from build123d import *

# Parameters (mm, degrees)
F1_DEPTH = 25.4
F2_T     = -5.08
F3_SIZE  = 10.16
F4_R     = 10.16
F5_R     = 15.875
F6_DEPTH = 25.4


with BuildPart() as f1:
    # F0 (on Top) → F1 (new body)
    with BuildSketch(Plane.XY):
        Polygon((25.4, 43.9940905122), (-25.4, 43.9940905122), (-50.8, 0), (-25.4, -43.9940905122), (25.4, -43.9940905122), (50.8, 0), align=None)
    extrude(amount=F1_DEPTH)

    # F2
    f2_openings = [f1.faces().sort_by_distance(p)[0] for p in [
        (0, 0, 25.4),
    ]]
    offset(amount=F2_T, openings=f2_openings)

    # F3
    f3_edges = [f1.edges().sort_by_distance(p)[0] for p in [
        (0, 38.914091, 5.08),
        (33.700591, 19.457045, 5.08),
        (-33.700591, 19.457045, 5.08),
        (-33.700591, -19.457045, 5.08),
        (0, -38.914091, 5.08),
        (33.700591, -19.457045, 5.08),
    ]]
    chamfer(f3_edges, length=F3_SIZE)

    # F4
    f4_edges = [f1.edges().sort_by_distance(p)[0] for p in [
        (0, 28.754091, 5.08),
        (24.901773, 14.377045, 5.08),
        (-24.901773, 14.377045, 5.08),
        (24.901773, -14.377045, 5.08),
        (-24.901773, -14.377045, 5.08),
        (0, -28.754091, 5.08),
    ]]
    fillet(f4_edges, radius=F4_R)

    # F5 (on face) → F6 (cut)
    with BuildSketch(Plane.XY.offset(5.08)):
        Circle(F5_R)
    extrude(amount=-F6_DEPTH, mode=Mode.SUBTRACT)


solid = f1.part
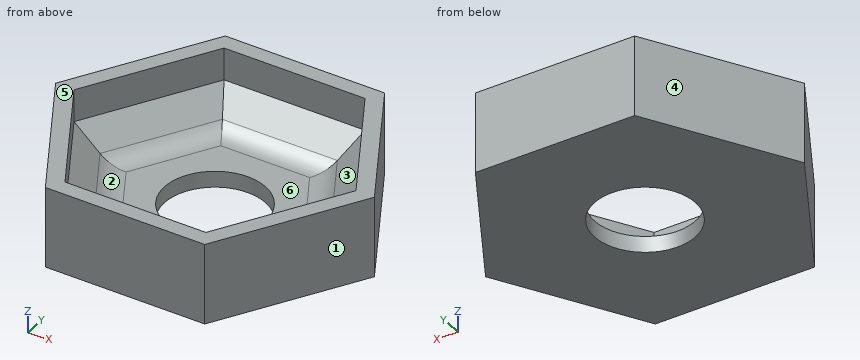
Geometry: final body of the model. Coordinates: model frame, mm. Face numbers are marked on the shaded views. A direction names the side the tool comes from. Coordinates: 2 decimals unless noted, no trailing zeros. Write each loop counter-clockwise with the first axis right and the second up, starting at its lowest first coordinate (ties: lowest second). Pieces come first, ordered by that corner, then holes. Notation, with made-up numbers: (84, 89.25) - (122, 89.25) arc R33 cw to (122, 128.25) - close; hole circle Ø3 at (63, -1). An arc over 180 degrees is marked (long way). Return JSON: item names as keys, results as strings.
Item 1: Section query C-C (y = -36). Output: boundary loops of the cut face in (x, z), and give its area (3 significant figures).
Completed:
{"outline": "(-30.02, 0) - (30.02, 0) - (30.02, 25.4) - (24.15, 25.4) - (24.15, 15.24) - (20.78, 12.33) - (-20.78, 12.33) - (-24.15, 15.24) - (-24.15, 25.4) - (-30.02, 25.4) - close", "area": "903 mm2"}
Item 2: Pull-direction query (X, two-part tool) for the marked faces 3, 4, 5 and 6; classes: +X half, -X half, draft (parallel to the pull), parting line (faces both ways), or undercut.
Completed:
{"face 3": "undercut", "face 4": "-X half", "face 5": "draft", "face 6": "undercut"}
Item 3: Section query D-D (x = 38). Output: boundary loops of the cut face in (y, z).
Completed:
{"outline": "(-22.17, 0) - (22.17, 0) - (22.17, 25.4) - (12.01, 25.4) - (12.01, 15.24) - (0, 9.23) - (-12.01, 15.24) - (-12.01, 25.4) - (-22.17, 25.4) - close"}
Item 4: Line query: L1, parallel to Y at x = 0, z = 2.1 (3 decimals); L2, parallel to Y at x = 13, z = 22.5; L3, parallel to X at y = 27, z = 20.25. Output: solid intervals per line, ascending.
Completed:
{"L1": "y = -43.994 to -15.875, 15.875 to 43.994", "L2": "y = -43.99 to -38.91, 38.91 to 43.99", "L3": "x = -35.21 to -29.35, 29.35 to 35.21"}
Item 5: Reachability of the marked faces 1 and 2 from +Z, -Z, +X, -X, +Y, -Y: full face, straight path, thin tool, end or side. Return the list, or none.
Completed:
{"face 1": "+Z, -Z, +X, -Y", "face 2": "+Z"}
Item 6: Section query B-B (z = 19.5). Output: boundary loops of the cut face in (x, y), and give its area (3 significant figures).
Completed:
{"outline": "(-50.8, 0) - (-25.4, -43.99) - (25.4, -43.99) - (50.8, 0) - (25.4, 43.99) - (-25.4, 43.99) - close; hole (-44.93, 0) - (-22.47, -38.91) - (22.47, -38.91) - (44.93, 0) - (22.47, 38.91) - (-22.47, 38.91) - close", "area": "1,460 mm2"}
Item 7: Section query A-A (x = 0). Output: boundary loops of the cut face in (y, z) (3 decimals).
Completed:
{"outline": "(-43.994, 0) - (-15.875, 0) - (-15.875, 5.08) - (-24.546, 5.08) arc R10.16 cw to (-31.73, 8.056) - (-38.914, 15.24) - (-38.914, 25.4) - (-43.994, 25.4) - close; (15.875, 0) - (43.994, 0) - (43.994, 25.4) - (38.914, 25.4) - (38.914, 15.24) - (31.73, 8.056) arc R10.16 cw to (24.546, 5.08) - (15.875, 5.08) - close"}
Item 8: Pin query (flat end, axial travel): pin 1 Ø19 at (x, y) = (0, 0) entering from -Z; pin 2 Ø24.5 at (x, y) = (-4.5, -0.5) entering from +Z; pin 3 Ø5 at (y, z) = (6.5, 7) entering from +X; pin 4 Ø4 at (y, z) = (5, 9.5) entering from +X. Return the tip coordinate at first contact, or that it passes through.
Completed:
{"pin 1": "passes through", "pin 2": "stops at z = 5.08", "pin 3": "stops at x = 48.49", "pin 4": "stops at x = 49.07"}
